For this review, use the dimensioned drawing (mm, ordinates from the lowest corner) and the shaded views. A direction names the side the tool comes from. Coordinates: 2 decimals unless noted, no trailing zeros. Write each loop counter-clockwise with the first axis right and the second up, starting at its lowest first coordinate (ties: lowest second). Pieces come first, ordered by that corner, then holes. Notation, with made-up numbers: (-11.75, 40) -> (11.25, 40) arc R25 cw to (11.25, 63) -> close; hole circle Ø8 at (-27.5, 50). An arc over 180 degrees is marked (long way). Return JSON: item names as keys, results as strings. Group by question number.
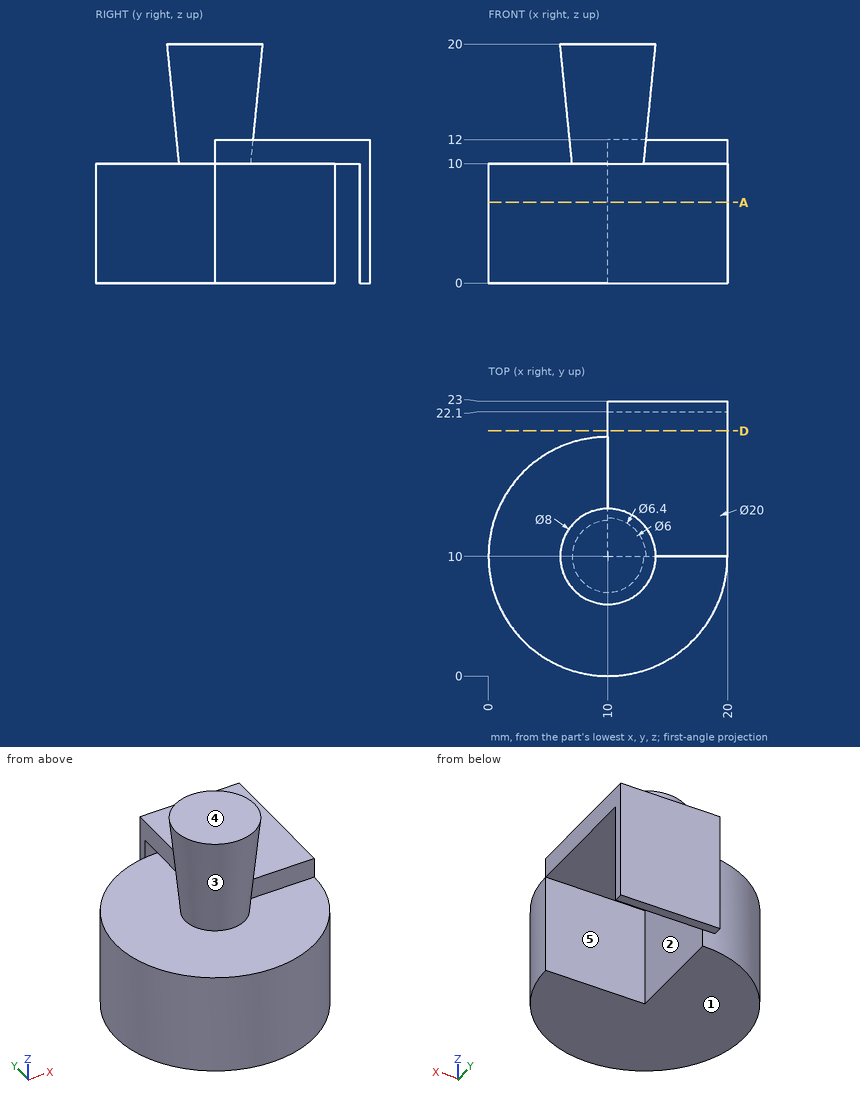
Q1. Wall thickness on L1, parallel to Z at x = 11, y = 11; L2, parallel to Z at x = 17, y = 3.75; L3, parallel to Y at x = 17.75, z = 5.5: over which ranges is each line inside the solid? List them lowest first.
Q2. We need section D-D on y = 20.5. Write out the cut boundary in (x, z).
Q3. For P1, Ø1, axis at x = 5.5, y = 5.5, coming from the +Z side; P2, Ø8, axis at x = 12.5, y = 14, coming from the +Z side; P3, Ø1, axis at x = 15, z = 11.5, coming from the -Y side; P4, Ø3, axis at x = 15.5, y = 13.5, coming from the +Z side, all flat-tipped, find the tip position at first contact; note any pin that passes through.
Q4. The part is to be moulded in two halves that separate along Z. For the marked faces 1, 2 and 3, say which applies: +Z half, -Z half, draft (parallel to the pull), parting line (faces both ways), or undercut.
Q5. We need section A-A on z = 6.75. Write out the cut boundary in (x, y).
Q6. For the marked faces 4 and 5, list the 3-axis set-ups (+Z, -Z, +X, -X, +Y, -Y) from which the entire face can be reached by the end or side of a thin tool; tool diameter is ignored.
Findings below:
{
 "1": {"L1": "z = 10 to 20", "L2": "z = 0 to 10", "L3": "y = 3.68 to 10, 22.1 to 23"},
 "2": {"outline": "(10, 10) -> (20, 10) -> (20, 12) -> (10, 12) -> close"},
 "3": {"P1": "stops at z = 10", "P2": "stops at z = 20", "P3": "stops at y = 10", "P4": "stops at z = 12"},
 "4": {"face 1": "-Z half", "face 2": "draft", "face 3": "undercut"},
 "5": {"outline": "(10, 10) -> (10, 20) arc R10 ccw (long way) to (20, 10) -> close; (10, 22.1) -> (20, 22.1) -> (20, 23) -> (10, 23) -> close"},
 "6": {"face 4": "+Z, +X, -X, +Y, -Y", "face 5": "-Z, +X"}
}
